Geometry: final body of the model. Coordinates: model frame, mm. A direction names the side the tool comes from. Round coordinates to 2 decimals unless told otherwise and drop trailing zeros. Write each loop counter-clockwise with the first axis right and the second up, starting at its lowest first coordinate (ties: lowest second). Pieces come first, ordered by that corner, then holes. Notation, with made-up numbers: M -6.5,36 L 15.5,36 A17 ccw 15.5,41 Z; hole C 76.5,-3.75 d4. An arc over 180 degrees is marked long. Use one line per item in the form item = value. Start each with the question number.
Autodesk Inventor part; units mm, degrees
ref_plane "YZ Plane" through (0, 0, 0) normal (1, 0, 0) x (0, 1, 0)
ref_plane "XZ Plane" through (0, 0, 0) normal (0, 1, 0) x (-1, 0, 0)
ref_plane "XY Plane" through (0, 0, 0) normal (0, 0, 1) x (1, 0, 0)
sketch "Sketch2" plane through (0, 0, 0) normal (0, 1, 0) x (-1, 0, 0)
  line L0 (381.1115, 61.7853) -> (30.3977, 61.7853)
  line L1 (380.9072, 412.5623) -> (381.1115, 61.7853)
  line L2 (30.1934, 412.5623) -> (380.9072, 412.5623)
  line L3 (30.3977, 61.7853) -> (30.3977, 412.5623)
  arc A0 (0.0977, 16.0853) -> (16.0601, 0.0853) centre (16.0335, 16.0213) ccw
  line L4 (0.0977, 16.0853) -> (-0.1066, 429.5623)
  arc A1 (15.8934, 445.5623) -> (-0.1066, 429.5623) centre (15.8934, 429.5623) ccw
  line L5 (15.8934, 445.5623) -> (395.2072, 445.5623)
  arc A2 (411.2072, 429.5623) -> (395.2072, 445.5623) centre (395.2072, 429.5623) ccw
  line L6 (411.2072, 429.5623) -> (411.4115, 16.0853)
  arc A3 (395.3739, 0.0853) -> (411.4115, 16.0853) centre (395.3472, 16.1497) ccw
  line L7 (395.3739, 0.0853) -> (16.0601, 0.0853)
  arc A4 (21.3351, 6.5853) -> (25.0851, 6.5853) centre (23.2101, 6.5853) ccw
  line L8 (25.0851, 10.5853) -> (25.0851, 6.5853)
  arc A5 (25.0851, 10.5853) -> (21.3351, 10.5853) centre (23.2101, 10.5853) ccw
  line L9 (21.3351, 6.5853) -> (21.3351, 10.5853)
  arc A6 (52.3351, 6.5853) -> (56.0851, 6.5853) centre (54.2101, 6.5853) ccw
  line L10 (56.0851, 10.5853) -> (56.0851, 6.5853)
  arc A7 (56.0851, 10.5853) -> (52.3351, 10.5853) centre (54.2101, 10.5853) ccw
  line L11 (52.3351, 6.5853) -> (52.3351, 10.5853)
  arc A8 (21.3351, 37.5853) -> (25.0851, 37.5853) centre (23.2101, 37.5853) ccw
  line L12 (25.0851, 41.5853) -> (25.0851, 37.5853)
  arc A9 (25.0851, 41.5853) -> (21.3351, 41.5853) centre (23.2101, 41.5853) ccw
  line L13 (21.3351, 37.5853) -> (21.3351, 41.5853)
  arc A10 (52.3351, 37.5853) -> (56.0851, 37.5853) centre (54.2101, 37.5853) ccw
  line L14 (56.0851, 41.5853) -> (56.0851, 37.5853)
  arc A11 (56.0851, 41.5853) -> (52.3351, 41.5853) centre (54.2101, 41.5853) ccw
  line L15 (52.3351, 37.5853) -> (52.3351, 41.5853)
  arc A12 (26.7101, 22.0853) -> (50.7101, 22.0853) centre (38.7101, 22.0853) ccw
  line L16 (50.7101, 26.0853) -> (50.7101, 22.0853)
  arc A13 (50.7101, 26.0853) -> (26.7101, 26.0853) centre (38.7101, 26.0853) ccw
  line L17 (26.7101, 22.0853) -> (26.7101, 26.0853)
  arc A14 (355.3489, 6.5853) -> (359.1299, 6.5853) centre (357.2394, 6.6008) ccw
  line L18 (359.1299, 10.5853) -> (359.1299, 6.5853)
  arc A15 (359.1299, 10.5853) -> (355.3489, 10.5853) centre (357.2394, 10.5698) ccw
  line L19 (355.3489, 6.5853) -> (355.3489, 10.5853)
  arc A16 (386.3313, 6.5853) -> (390.0989, 6.577) centre (388.215, 6.5376) ccw
  arc A17 (386.3384, 37.5853) -> (390.0884, 37.5853) centre (388.2134, 37.5853) ccw
  line L20 (390.0884, 41.5853) -> (390.0884, 37.5853)
  arc A18 (390.0884, 41.5853) -> (386.3384, 41.5853) centre (388.2134, 41.5853) ccw
  line L21 (386.3384, 37.5853) -> (386.3384, 41.5853)
  arc A19 (355.3298, 37.5853) -> (359.0798, 37.5853) centre (357.2048, 37.5853) ccw
  line L22 (359.0798, 41.5853) -> (359.0798, 37.5853)
  arc A20 (359.0798, 41.5853) -> (355.3489, 41.5853) centre (357.2143, 41.5948) ccw
  line L23 (355.3298, 37.5853) -> (355.3489, 41.5853)
  arc A21 (360.6847, 22.0853) -> (384.6847, 22.0853) centre (372.6847, 22.0853) ccw
  line L24 (384.6847, 26.0853) -> (384.6847, 22.0853)
  arc A22 (384.6847, 26.0853) -> (360.6847, 26.0853) centre (372.6847, 26.0853) ccw
  line L25 (360.6847, 22.0853) -> (360.6847, 26.0853)
  circle A23 centre (50.1434, 420.5623) radius 2.1
  circle A24 centre (38.5434, 435.5623) radius 2.1
  circle A25 centre (372.5572, 435.5623) radius 2.1
  circle A26 centre (360.9572, 420.5623) radius 2.1
  circle A27 centre (25.7809, 418.0623) radius 1.6
  circle A28 centre (66.7809, 418.0623) radius 1.6
  circle A29 centre (205.5503, 418.0623) radius 1.6
  circle A30 centre (344.3197, 418.0623) radius 1.6
  circle A31 centre (386.2129, 418.0623) radius 1.6
  circle A32 centre (385.3197, 56.2853) radius 1
  circle A33 centre (344.3197, 56.2853) radius 1
  circle A34 centre (205.5503, 56.2853) radius 1
  circle A35 centre (66.7809, 56.2853) radius 1
  circle A36 centre (25.7809, 56.2853) radius 1
  arc A37 (390.0989, 10.5853) -> (386.3489, 10.5853) centre (388.2239, 10.5853) ccw
  line L26 (378.8199, 179.5488) -> (32.1952, 179.5488)
  circle A38 centre (60.6452, 222.8238) radius 1.6
  circle A39 centre (60.6452, 258.6363) radius 1.6
  circle A40 centre (60.6452, 187.0113) radius 1.6
  circle A41 centre (350.3699, 187.0113) radius 1.6
  circle A42 centre (350.3699, 222.8238) radius 1.6
  circle A43 centre (350.3699, 258.6363) radius 1.6
  circle A44 centre (49.8452, 185.8988) radius 1.6
  circle A45 centre (49.8452, 259.7488) radius 1.6
  circle A46 centre (361.1699, 222.8238) radius 1.6
  line L27 (378.8199, 266.0988) -> (378.8199, 179.5488)
  line L28 (345.8699, 256.5738) -> (345.8699, 189.0738)
  line L29 (65.1452, 256.5738) -> (345.8699, 256.5738)
  line L30 (65.1452, 189.0738) -> (65.1452, 256.5738)
  line L31 (345.8699, 189.0738) -> (65.1452, 189.0738)
  line L32 (32.1952, 179.5488) -> (32.1952, 266.0988)
  line L33 (32.1952, 266.0988) -> (378.8199, 266.0988)
  circle A47 centre (50.1452, 204.5238) radius 2.1
  circle A48 centre (360.8699, 204.5238) radius 2.1
  circle A49 centre (360.8699, 241.1238) radius 2.1
  circle A50 centre (50.1452, 241.1238) radius 2.1
  line L34 (224.6003, 203.7738) -> (186.5003, 203.7738)
  line L35 (224.6003, 207.8328) -> (224.6003, 203.7738)
  arc A51 (226.0103, 209.3301) -> (224.6003, 207.8328) centre (226.1003, 207.8328) ccw
  arc A52 (226.0103, 209.3301) -> (226.0103, 216.3175) centre (225.8003, 212.8238) ccw
  arc A53 (224.6003, 217.8148) -> (226.0103, 216.3175) centre (226.1003, 217.8148) ccw
  arc A54 (226.0103, 229.3301) -> (224.6003, 227.8328) centre (226.1003, 227.8328) ccw
  arc A55 (226.0103, 229.3301) -> (226.0103, 236.3175) centre (225.8003, 232.8238) ccw
  arc A56 (224.6003, 237.8148) -> (226.0103, 236.3175) centre (226.1003, 237.8148) ccw
  line L36 (186.5003, 241.8738) -> (224.6003, 241.8738)
  line L37 (186.5003, 237.8148) -> (186.5003, 241.8738)
  arc A57 (185.0903, 236.3175) -> (186.5003, 237.8148) centre (185.0003, 237.8148) ccw
  arc A58 (185.0903, 236.3175) -> (185.0903, 229.3301) centre (185.3003, 232.8238) ccw
  arc A59 (186.5003, 227.8328) -> (185.0903, 229.3301) centre (185.0003, 227.8328) ccw
  arc A60 (185.0903, 216.3175) -> (186.5003, 217.8148) centre (185.0003, 217.8148) ccw
  arc A61 (185.0903, 216.3175) -> (185.0903, 209.3301) centre (185.3003, 212.8238) ccw
  arc A62 (186.5003, 207.8328) -> (185.0903, 209.3301) centre (185.0003, 207.8328) ccw
  line L38 (173.8003, 254.5738) -> (237.3003, 254.5738)
  line L39 (237.3003, 254.5738) -> (237.3003, 191.0738)
  line L40 (237.3003, 191.0738) -> (173.8003, 191.0738)
  line L41 (173.8003, 191.0738) -> (173.8003, 254.5738)
  circle A63 centre (180.1503, 197.0113) radius 0.875
  circle A64 centre (230.9503, 197.0113) radius 0.875
  circle A65 centre (230.9503, 248.6363) radius 0.875
  circle A66 centre (180.1503, 248.6363) radius 0.875
  circle A67 centre (177.8003, 232.8238) radius 0.875
  circle A68 centre (233.3003, 232.8238) radius 0.875
  circle A69 centre (233.3003, 212.8238) radius 0.875
  circle A70 centre (177.8003, 212.8238) radius 0.875
  line L42 (186.5003, 203.7738) -> (186.5003, 207.8328)
  line L43 (186.5003, 217.8148) -> (186.5003, 227.8328)
  line L44 (224.6003, 241.8738) -> (224.6003, 237.8148)
  line L45 (224.6003, 227.8328) -> (224.6003, 217.8148)
  line L46 (390.0989, 10.5853) -> (390.0989, 6.577)
  line L47 (386.3489, 10.5853) -> (386.3313, 6.5853)
  circle A71 centre (136.7809, 56.2853) radius 1
  circle A72 centre (273.8132, 56.2853) radius 1
  circle A73 centre (274.3197, 418.0623) radius 1.6
  circle A74 centre (136.7809, 418.0623) radius 1.6
  point P0 (0, 0)
extrude "Extrusion1" add sketch "Sketch2" along normal blind 4 contours L4 A1 L5 A2 L6 A3 L7 A0
properties part number "300 mm top plate"
1. Section query B-B (z = 237). Return loops of the section in (x, y).
2. Ray query, probe 1 along Z at (x, y) = (-42.5, 2.95); probe 2 along Z at (x, y) = (-259, 0.4); probe 3 along X at (y, z) = (2.65, 181). Return the intervals inside material, ascending.
3. Contact query for flat-ended pins moving along their axis: pin 1 (1.2 mm diameter, centred on y = 2, z = 9.5, fed in from +X); pin 2 (1.2 mm diameter, centred on y = 2, z = 8, fed in from -X); pin 3 (2 mm diameter, centred on y = 2, z = 39.5, fed in from +X). Output: stop coordinate, or through.
4. Section query C-C (y = 1.2). Give the number of separate pieces and of enclosed holes in the cut face, then the cut area to 3 significant figures.
5. Set-up query: faces 1 (the face through (-406.396, 1.972, 441)), 2 (the face through (-372.421, 1.972, 38.082)). Return all of +Z, -Z, +X, -X, +Y, -Y with unobstructed straight access to the full face (end or side cutting, diameter ignored); none if empty.
6. Section query A-A (x = -265.5). Return loops of the section in (y, z).
7. Pull-direction query (Z, two-part tool) for faces 3 (the face through (-20, 4, 226)), 4 (the face through (-38.446, 1.972, 38.082)), 5 (the face through (-406.817, 1.972, 4.902)); classes: released by +Z, released by -Z, zero draft, split by the parting line, or undercut.
Checks:
q1.outline = M -411.3,0 L -381.01,0 L -381.01,4 L -411.3,4 Z; M -30.4,0 L 0.01,0 L 0.01,4 L -30.4,4 Z
q2.probe_1 = 0.09 to 10.7, 37.47 to 61.79, 412.56 to 445.56
q2.probe_2 = 0.09 to 61.79, 412.56 to 445.56
q2.probe_3 = -411.33 to -381.04, -30.4 to -0.02
q3.pin_1 = -1.24
q3.pin_2 = -409.53
q3.pin_3 = -0.09
q4.separate_pieces = 1
q4.enclosed_holes = 29
q4.area = 58,600 mm^2
q5.face_1 = +Z, -X, +Y, -Y
q5.face_2 = +Y, -Y
q6.outline = M 0,0.09 L 4,0.09 L 4,61.79 L 0,61.79 Z; M 0,412.56 L 4,412.56 L 4,445.56 L 0,445.56 Z
q7.face_3 = zero draft
q7.face_4 = undercut
q7.face_5 = released by -Z
